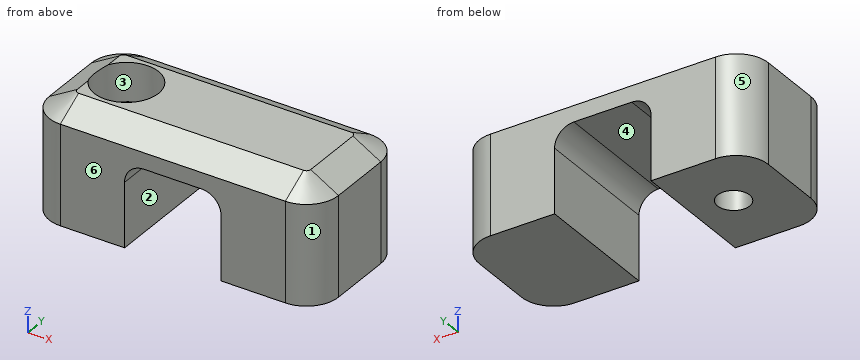
from build123d import *

# Parameters (mm, degrees)
SKETCH1_W       = 45
SKETCH1_H       = 20
EXTRUDE1_DEPTH  = 5
SKETCH2_W       = 15
SKETCH2_H       = 20
EXTRUDE2_DEPTH  = 13
SKETCH3_R       = 5
EXTRUDE3_DEPTH  = 6
SKETCH4_R       = 2.5
EXTRUDE4_DEPTH  = 16
FILLET1_R       = 5
CHAMFER1_SIZE   = 4.330127019
CHAMFER1_SIZE_2 = 2.5
FILLET2_R       = 3
FILLET3_R       = 3


with BuildPart() as part:
    # Sketch1 → Extrude1 (new body)
    with BuildSketch(Plane.XY):
        Rectangle(SKETCH1_W, SKETCH1_H)
    extrude(amount=EXTRUDE1_DEPTH)

    # Sketch2 → Extrude2 (add)
    with BuildSketch(Plane(origin=(0, 0, 0), x_dir=(-1, 0, 0), z_dir=(0, 0, -1))):
        with Locations((15, 0)):
            Rectangle(SKETCH2_W, SKETCH2_H)
        with Locations((-15, 0)):
            Rectangle(SKETCH2_W, SKETCH2_H)
    extrude(amount=EXTRUDE2_DEPTH)

    # Sketch3 → Extrude3 (cut)
    with BuildSketch(Plane.XY.offset(5)):
        with Locations((-13.77840955, 0)):
            Circle(SKETCH3_R)
    extrude(amount=-EXTRUDE3_DEPTH, mode=Mode.SUBTRACT)

    # Sketch4 → Extrude4 (cut)
    with BuildSketch(Plane.XY.offset(-1)):
        with Locations((-13.77840955, 0)):
            Circle(SKETCH4_R)
    extrude(amount=-EXTRUDE4_DEPTH, mode=Mode.SUBTRACT)

    # Fillet1
    fillet1_edges = [part.edges().sort_by_distance(p)[0] for p in [
        (-22.5, 10, -4),
        (22.5, 10, -4),
        (22.5, -10, -4),
        (-22.5, -10, -4),
    ]]
    fillet(fillet1_edges, radius=FILLET1_R)

    # Chamfer1
    # the kernel refuses this chamfer: 4.330127019, 2.5 mm, written as the material it takes off along each edge
    with BuildSketch(Plane(origin=(22.5, 5, 5), x_dir=(-0.999813220622208, 0, 0.01932676561270069), z_dir=(0, -1, 0)), Plane(origin=(-22.5, -5, 5), x_dir=(0.999813220622208, 0, 0.01932676561270069), z_dir=(0, 1, 0))) as chamfer1_piece_1:
        Polygon((CHAMFER1_SIZE * 0.999813220604, CHAMFER1_SIZE * 0.0193267656124), (-CHAMFER1_SIZE_2 * 0.0193267656127, CHAMFER1_SIZE_2 * 0.999813220622), (0, 0), align=None)
    extrude(amount=10, mode=Mode.SUBTRACT)
    with BuildSketch(Plane(origin=(17.5, -10, 5), x_dir=(0, -0.05789386240267114, -0.9983227437537926), z_dir=(-1, 0, 0))) as chamfer1_piece_2:
        Polygon((CHAMFER1_SIZE_2 * 0.998322743754, -CHAMFER1_SIZE_2 * 0.0578938624027), (-CHAMFER1_SIZE * 0.0578938624016, -CHAMFER1_SIZE * 0.998322743736), (0, 0), align=None)
    extrude(amount=35, mode=Mode.SUBTRACT)
    with BuildSketch(Plane(origin=(-17.5, 10, 5), x_dir=(0, -0.999813220622208, 0.01932676561270069), z_dir=(1, 0, 0))) as chamfer1_piece_3:
        Polygon((CHAMFER1_SIZE * 0.999813220604, CHAMFER1_SIZE * 0.0193267656124), (-CHAMFER1_SIZE_2 * 0.0193267656127, CHAMFER1_SIZE_2 * 0.999813220622), (0, 0), align=None)
    extrude(amount=35, mode=Mode.SUBTRACT)
    with BuildSketch(Plane(origin=(-17.5, 5, 5), x_dir=(-1, 0, 0), z_dir=(0, -1, 0))) as chamfer1_piece_4:
        Polygon((5 - CHAMFER1_SIZE, 0), (5, CHAMFER1_SIZE_2), (5, 0), align=None)
    revolve(axis=Axis((-17.5, 5, 5), (0, 0, -1)), revolution_arc=90, mode=Mode.SUBTRACT)
    with BuildSketch(Plane(origin=(-17.5, -5, 5), x_dir=(0, -1, 0), z_dir=(1, 0, 0))) as chamfer1_piece_5:
        Polygon((5 - CHAMFER1_SIZE, 0), (5, CHAMFER1_SIZE_2), (5, 0), align=None)
    revolve(axis=Axis((-17.5, -5, 5), (0, 0, -1)), revolution_arc=90, mode=Mode.SUBTRACT)
    with BuildSketch(Plane(origin=(17.5, 5, 5), x_dir=(1, 0, 0), z_dir=(0, -1, 0))) as chamfer1_piece_6:
        Polygon((5 - CHAMFER1_SIZE, 0), (5, -CHAMFER1_SIZE_2), (5, 0), align=None)
    revolve(axis=Axis((17.5, 5, 5), (0, 0, 1)), revolution_arc=90, mode=Mode.SUBTRACT)
    with BuildSketch(Plane(origin=(17.5, -5, 5), x_dir=(0, -1, 0), z_dir=(-1, 0, 0))) as chamfer1_piece_7:
        Polygon((5 - CHAMFER1_SIZE, 0), (5, -CHAMFER1_SIZE_2), (5, 0), align=None)
    revolve(axis=Axis((17.5, -5, 5), (0, 0, 1)), revolution_arc=90, mode=Mode.SUBTRACT)

    # Fillet2
    fillet2_edges = [part.edges().sort_by_distance(p)[0] for p in [
        (-7.5, 0, 0),
    ]]
    fillet(fillet2_edges, radius=FILLET2_R)

    # Fillet3
    fillet3_edges = [part.edges().sort_by_distance(p)[0] for p in [
        (7.5, 0, 0),
    ]]
    fillet(fillet3_edges, radius=FILLET3_R)


solid = part.part
Work out the finished part from the listing and answer in its coordinate system (mm). Face numbers are marked on the shaded views. A direction names the side the tool comes from. Give positions to 0.01 mm unless a question says otherwise; leave off trailing zeros. Loops run counter-clockwise (first coordinate to the right, second up) from the corner with the lowest first, then second, coordinate; pieces in that order, holes last. Notation, with made-up numbers: (32, -0.75) - (67, -0.75) arc R32 cw to (67, 26.25) - close; hole circle Ø7 at (51, -3). An arc over 180 degrees is marked (long way). Answer in a Markdown table with one row per item. Add a question column.
Q1. Determine the mould class of the marked faces 4, 5 and 6 for opening direction X: released by +X, released by -X, zero draft, split by the parting line, or undercut.
Q2. The part is cut by section B-B (z = 1.5). Determine the outline of the cut face in (x, y).
Q3. This flat-tipped pin is pushed along its axis until it touches: P1, Ø10, axis at x = 0, y = 4.5, coming from the -Z side. Where does it stop, or does it pass through?
Q4. The part is cut by section D-D (x = 11.5). Determine the outline of the cut face in (y, z).
Q5. The part is cut by section A-A (z = -10.25). Determine the outline of the cut face in (x, y).
Q6. The part is cut by section C-C (y = 0). Determine the outline of the cut face in (x, z), and give its area (3 significant figures).
Q7. A tool of negligible diameter and unlimited length cuts with its end or side. For the marked faces 1, 2 and 3, from which of +Z, -Z, +X, -X, +Y, -Y can it reach the whole face along a straight path? Write none if from no direction.
Q8. Consider line 1 along X through (y, z) = (0, 0.85); line 2 along X through (y, z) = (5.5, -3.75); line 3 along Y through (x, z) = (-16, 3). Determine where each line is inside the solid, lowest interval first.
Solution:
| question | item | result |
|---|---|---|
| 1 | face 4 | undercut |
| 1 | face 5 | released by -X |
| 1 | face 6 | zero draft |
| 2 | outline | (-22.5, -5) arc R5 ccw to (-17.5, -10) - (17.5, -10) arc R5 ccw to (22.5, -5) - (22.5, 5) arc R5 ccw to (17.5, 10) - (-17.5, 10) arc R5 ccw to (-22.5, 5) - close; hole circle Ø10 at (-13.78, 0) |
| 3 | P1 | stops at z = -0.04 |
| 4 | outline | (-10, -13) - (10, -13) - (10, 2.5) - (5.67, 5) - (-5.67, 5) - (-10, 2.5) - close |
| 5 | outline | (-22.5, -5) arc R5 ccw to (-17.5, -10) - (-7.5, -10) - (-7.5, 10) - (-17.5, 10) arc R5 ccw to (-22.5, 5) - close; (7.5, -10) - (17.5, -10) arc R5 ccw to (22.5, -5) - (22.5, 5) arc R5 ccw to (17.5, 10) - (7.5, 10) - close; hole circle Ø5 at (-13.78, 0) |
| 6 | outline | (-22.5, -13) - (-16.28, -13) - (-16.28, -1) - (-18.78, -1) - (-18.78, 4.65) - (-22.5, 2.5) - close; (-11.28, -13) - (-7.5, -13) - (-7.5, -3) arc R3 cw to (-4.5, 0) - (4.5, 0) arc R3 cw to (7.5, -3) - (7.5, -13) - (22.5, -13) - (22.5, 2.5) - (18.17, 5) - (-8.78, 5) - (-8.78, -1) - (-11.28, -1) - close |
| 6 | area | 488 mm² |
| 7 | face 1 | +Z, -Z, +X, -Y |
| 7 | face 2 | -Z, +Y, -Y |
| 7 | face 3 | +Z |
| 8 | line 1 | x = -22.5 to -18.78, -8.78 to 22.5 |
| 8 | line 2 | x = -22.47 to -7.5, 7.5 to 22.47 |
| 8 | line 3 | y = -9.13 to -4.48, 4.48 to 9.13 |
